Input: part model. Units: mm. Frame: model coordinates. Face numbers are marked on the shaded views. A direction names the side the tool comes from. Give positions to 0.01 mm unless a question says otherwise; leave off trailing zeros. Loops run counter-clockwise (first coordinate to the right, second up) from the corner with the lowest first, then second, coordinate; pieces in that order, holes last. Notation, with made-up numbers: (76, 19.5) - (121, 19.5) arc R11 ccw to (121, 40.5) - close; hole circle Ø4 at (-22, -27.75). An arc over 180 degrees is marked (long way). Answer as a JSON object with one key per item and string values. Group by question number.
(1) Section query B-B (y = -12). Return loops of the section in (x, z), plus the area to 3 significant figures.
(2) Section query C-C (z = 9). Return loops of the section in (x, y), plus the area to 3 significant figures.
(3) Mould query, pull axis Z, two halves, no side actions, for the marked faces 1, 2 and 3. Classes: +Z half, -Z half, draft (parallel to the pull), parting line (faces both ways), or undercut.
(4) Access query for the marked faces 4 and 5. Directions: +Z, -Z, +X, -X, +Y, -Y. A direction counts if a zero-diameter tool reaches every point of the face in a straight line with its end or side. Return the directions, or none.
(5) Pin query (flat end, axial travel): P1, Ø10, axis at x = 10, z = 61, coming from the -Y side. Return the tip coordinate at first contact, or that it passes through.
(6) Material intervals for L1, parallel to Z at x = -68, y = -49.5; L2, parallel to X at y = -42, z = 99; L3, parallel to Y at x = 49, z = -97, sorted ascending.
(7) Section query A-A (x = 59). Return loops of the section in (y, z), plus the area to 3 significant figures.
```python
from build123d import *

# Parameters (mm, degrees)
F0_W     = 170
F0_H     = 232
F1_DEPTH = 67
F2_T     = -1
F3_R     = 1


with BuildPart() as f1:
    # F0 (on Front) → F1 (new body)
    with BuildSketch(Plane.XZ):
        Rectangle(F0_W, F0_H)
    extrude(amount=F1_DEPTH)

    # F2
    f2_openings = [f1.faces().sort_by_distance(p)[0] for p in [
        (0, -67, 0),
    ]]
    offset(amount=F2_T, openings=f2_openings)

    # F3
    f3_edges = [f1.edges().sort_by_distance(p)[0] for p in [
        (85, -33.5, -116),
        (85, -33.5, 116),
        (85, 0, 0),
        (0, 0, -116),
        (-85, 0, 0),
        (-85, -33.5, -116),
        (-85, -33.5, 116),
        (0, 0, 116),
        (84, -34, 115),
        (0, -1, -115),
        (84, -1, 0),
        (0, -1, 115),
        (-84, -1, 0),
        (84, -34, -115),
        (-84, -34, 115),
    ]]
    fillet(f3_edges, radius=F3_R)


solid = f1.part
```
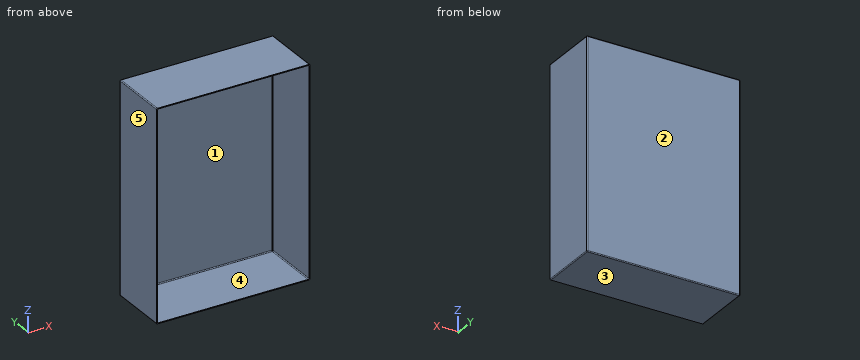
Recorded:
{
 "1": {"outline": "(-85, -115) arc R1 ccw to (-84, -116) - (84, -116) arc R1 ccw to (85, -115) - (85, 115) arc R1 ccw to (84, 116) - (-84, 116) arc R1 ccw to (-85, 115) - close; hole (-84, -115) - (83, -115) arc R1 ccw to (84, -114) - (84, 114) arc R1 ccw to (83, 115) - (-83, 115) arc R1 ccw to (-84, 114) - close", "area": "800 mm^2"},
 "2": {"outline": "(-85, -67) - (-84, -67) - (-84, -2) arc R1 cw to (-83, -1) - (83, -1) arc R1 cw to (84, -2) - (84, -67) - (85, -67) - (85, -1) arc R1 ccw to (84, 0) - (-84, 0) arc R1 ccw to (-85, -1) - close", "area": "302 mm^2"},
 "3": {"face 1": "undercut", "face 2": "draft", "face 3": "-Z half"},
 "4": {"face 4": "-Y", "face 5": "+Z, -Z, -X, +Y, -Y"},
 "5": {"P1": "stops at y = -1"},
 "6": {"L1": "z = -116 to -115, 115 to 116", "L2": "x = -85 to -84, 84 to 85", "L3": "y = -1 to 0"},
 "7": {"outline": "(-67, -116) - (-1, -116) arc R1 ccw to (0, -115) - (0, 115) arc R1 ccw to (-1, 116) - (-67, 116) - (-67, 115) - (-2, 115) arc R1 cw to (-1, 114) - (-1, -114) arc R1 cw to (-2, -115) - (-67, -115) - close", "area": "364 mm^2"}
}
